Verification items for the finished model (mm, model axes). A direction names the side the tool comes from. Round coordinates to 2 decimals unless told otherwise and drop trailing zeros. Order: outer loops, then holes, each group sorted by start corner. A loop starts at its lowest first (then second) coordinate and runs counter-clockwise, first axis right, second up. Notation, with made-up numbers: (88, 72) -> (105, 72) arc R21 cw to (105, 82) -> close; hole circle Ø8 at (55, -18.75). An arc over 180 degrees is marked (long way). Answer in a Markdown table with one row per item. Add a question column.
```python
from build123d import *

# Parameters (mm, degrees)
BOSS_EXTRUDE1_DEPTH = 7
BOSS_EXTRUDE2_DEPTH = 2
BOSS_EXTRUDE3_START = 2
SKETCH3_R           = 2.25
BOSS_EXTRUDE3_DEPTH = 1
CABLE_START         = -22.5
SKETCH6_R           = 1.75
CABLE_TUBES_DEPTH   = 20
WIRE_START          = -22.5
WIRE_CANALS_DEPTH   = 8
SKETCH4_R           = 0.8
SCREW_HOLES_DEPTH   = 8.0000001
CUT_EXTRUDE2_START  = 3
CUT_EXTRUDE2_DEPTH  = 4


with BuildPart() as part:
    # Sketch1 → Boss-Extrude1 (new body)
    with BuildSketch(Plane.XY):
        with BuildLine():
            Line((14.142135624, -14.142135624), (11.313708499, -11.313708499))
            ThreePointArc((11.313708499, -11.313708499), (-3.056276198, -15.70538684), (-14.730729168, -6.245447796))
            Line((-14.730729168, -6.245447796), (-22.627416999, -14.142135627))
            Line((-22.627416999, -14.142135627), (-19.091883095, -17.677669532))
            Line((-19.091883095, -17.677669532), (-14.849242408, -13.435028845))
            Line((-14.849242408, -13.435028845), (-9.899494939, -18.384776313))
            Line((-9.899494939, -18.384776313), (-14.142135626, -22.627417))
            Line((-14.142135626, -22.627417), (-10.60660172, -26.162950906))
            Line((-10.60660172, -26.162950906), (-6.443650814, -22))
            Line((-6.443650814, -22), (6.284271247, -22))
            Line((6.284271247, -22), (14.142135624, -14.142135624))
        make_face()
    extrude(amount=BOSS_EXTRUDE1_DEPTH)

    # Sketch2 → Boss-Extrude2 (add)
    with BuildSketch(Plane.XY):
        with BuildLine():
            Line((-2.5, 0), (-2.5, -22))
            Line((-2.5, -22), (2.5, -22))
            Line((2.5, -22), (2.5, 0))
            ThreePointArc((2.5, 0), (0, 2.5), (-2.5, 0))
        make_face()
    extrude(amount=BOSS_EXTRUDE2_DEPTH)

    # Sketch3 → Boss-Extrude3 (add)
    with BuildSketch(Plane.XY.offset(BOSS_EXTRUDE3_START)):
        Circle(SKETCH3_R)
    extrude(amount=BOSS_EXTRUDE3_DEPTH)

    # Sketch6 → Cable Tubes (cut)
    with BuildSketch(Plane(origin=(0, 0, 0), x_dir=(1, 0, 0), z_dir=(0, 1, 0)).offset(CABLE_START)):
        with Locations((-4, -7)):
            Circle(SKETCH6_R)
        with Locations((4, -7)):
            Circle(SKETCH6_R)
    extrude(amount=CABLE_TUBES_DEPTH, mode=Mode.SUBTRACT)

    # Sketch7 → Wire Canals (cut)
    with BuildSketch(Plane(origin=(0, 0, 0), x_dir=(1, 0, 0), z_dir=(0, 1, 0)).offset(WIRE_START)):
        Polygon((-3, -7), (3, -7), (3, -6), (2, -6), (2, -4), (-2, -4), (-2, -6), (-3, -6), align=None)
    extrude(amount=WIRE_CANALS_DEPTH, mode=Mode.SUBTRACT)

    # Sketch4 → Screw Holes (cut, through all)
    with BuildSketch(Plane.XY):
        with Locations((-11.318596704, -23.329658004)):
            Circle(SKETCH4_R)
        with Locations((-17.682557735, -12.723056286)):
            Circle(SKETCH4_R)
        with Locations((8, -17)):
            Circle(SKETCH4_R)
        with Locations((-9.197276361, -21.20833766)):
            Circle(SKETCH4_R)
        with Locations((-8, -17)):
            Circle(SKETCH4_R)
        with Locations((-19.803878078, -14.84437663)):
            Circle(SKETCH4_R)
    extrude(amount=SCREW_HOLES_DEPTH, mode=Mode.SUBTRACT)

    # Sketch10 → Cut-Extrude2 (cut)
    with BuildSketch(Plane.XY.offset(CUT_EXTRUDE2_START)):
        Polygon((-19.091883095, -17.677669532), (-14.849242408, -13.435028845), (-18.384776312, -9.89949494), (-22.627416999, -14.142135627), align=None)
        Polygon((-14.142135626, -22.627417), (-9.899494939, -18.384776313), (-6.284271253, -22), (-6.443650814, -22), (-10.60660172, -26.162950906), align=None)
    extrude(amount=CUT_EXTRUDE2_DEPTH, mode=Mode.SUBTRACT)


solid = part.part
```
1) Thickness scan on L1, parallel to Y at x = -12, z = 0.5; L2, parallel to X at y = -14, z = 0.75; L3, parallel to X at y = -14.25, z = 2.75. Record the ranges inside material, lowest first. Write a range as [from, to].
2) Tool access check on faces 1 (the face through (-2.5, -8, 1)), 2 (the face through (-17, -15.586, 1.479)), 3 (the face through (0, -19, 4)). Record the directions out of +Z, -Z, +X, -X, +Y, -Y that give a thin tool (end or side, any length) a straight path to the whole face; none if there is none.
3) Cross-section at B-B, the plane y = -17. Record the boundary of the cut face in (x, z).
4) Draft check along X on faces 4 (the face through (-0.29, 2.23, 2.49)), 5 (the face through (-8.554, -24.111, 1.479)), 6 (the face through (0, 0, 3)), 7 (the face through (2, -19, 5)). Enter one of: +X half, -X half, draft (parallel to the pull), parting line (faces both ways), or undercut.
5) Cross-section at D-D, the plane y = -5. Record the boundary of the cut face in (x, z), and give its area (3 significant figures).
6) Cross-section at A-A, the plane x = 0. Record the boundary of the cut face in (y, z), and give its area (3 significant figures).
7) Cross-section at C-C, the plane x = 8. Record the boundary of the cut face in (y, z).
8) Depth check by flat-ended pin: P1, Ø1.4, axis at x = 8, y = -17, coming from the +Z side; P2, Ø1.5, axis at x = -1, y = -3, coming from the +Z side; P3, Ø0.6, axis at x = -2, y = -19, coming from the +Z side; P4, Ø1, axis at y = -12.5, z = 2.5, coming from the +X side. Enter the tip coordinate at first touch or a pass-through.
Results below:
| question | item | result |
|---|---|---|
| 1 | L1 | [-24.77, -23.75], [-22.91, -20.49], [-16.28, -10.58] |
| 1 | L2 | [-22.49, -15.41], [-14.28, -7.75], [-2.5, 2.5], [7.75, 14] |
| 1 | L3 | [-22.52, -20.34], [-19.27, -15.66], [-14.03, -7.28], [7.28, 14.03] |
| 2 | face 1 | +Z, -Z, +Y |
| 2 | face 2 | +Z, -Z, -Y |
| 2 | face 3 | +Z, +Y, -Y |
| 3 | outline | (-19.77, 0) -> (-18.41, 0) -> (-18.41, 3) -> (-19.77, 3) -> close; (-11.28, 0) -> (-8.8, 0) -> (-8.8, 7) -> (-11.28, 7) -> close; (-7.2, 0) -> (7.2, 0) -> (7.2, 7) -> (5.75, 7) arc R1.75 cw to (2.56, 6) -> (2, 6) -> (2, 4) -> (-2, 4) -> (-2, 6) -> (-2.56, 6) arc R1.75 cw to (-5.75, 7) -> (-7.2, 7) -> close; (8.8, 0) -> (11.28, 0) -> (11.28, 7) -> (8.8, 7) -> close |
| 4 | face 4 | parting line |
| 4 | face 5 | +X half |
| 4 | face 6 | draft |
| 4 | face 7 | undercut |
| 5 | outline | (-2.5, 0) -> (2.5, 0) -> (2.5, 2) -> (-2.5, 2) -> close |
| 5 | area | 10.0 mm² |
| 6 | outline | (-22, 0) -> (2.5, 0) -> (2.5, 2) -> (2.25, 2) -> (2.25, 3) -> (-2.25, 3) -> (-2.25, 2) -> (-16, 2) -> (-16, 4) -> (-22, 4) -> close |
| 6 | area | 65.5 mm² |
| 7 | outline | (-20.28, 0) -> (-17.8, 0) -> (-17.8, 7) -> (-20.28, 7) -> close; (-16.2, 0) -> (-13.86, 0) -> (-13.86, 7) -> (-16.2, 7) -> close |
| 8 | P1 | through |
| 8 | P2 | z = 2 |
| 8 | P3 | z = 6 |
| 8 | P4 | x = 13 |
